The figure shows three views and two pictorial views of one solid part (mm, origin at its lowest corner). Answer the questions. A direction names the side the tool comes from. Give positions to 0.01 mm unless a question says otherwise; leave off trailing zeros. Order: outer loops, then holes, each group sorted by start corner. A loop starts at its lowest first (then second) coordinate and runs counter-clockwise, first axis right, second up. Notation, with made-up numbers: (49.25, 58.5) -> (62.25, 58.5) arc R18 ccw to (62.25, 91.5) -> close; hole circle Ø4 at (78.25, 54). An arc over 180 degrees is marked (long way). Use one line per item in the form item = value.
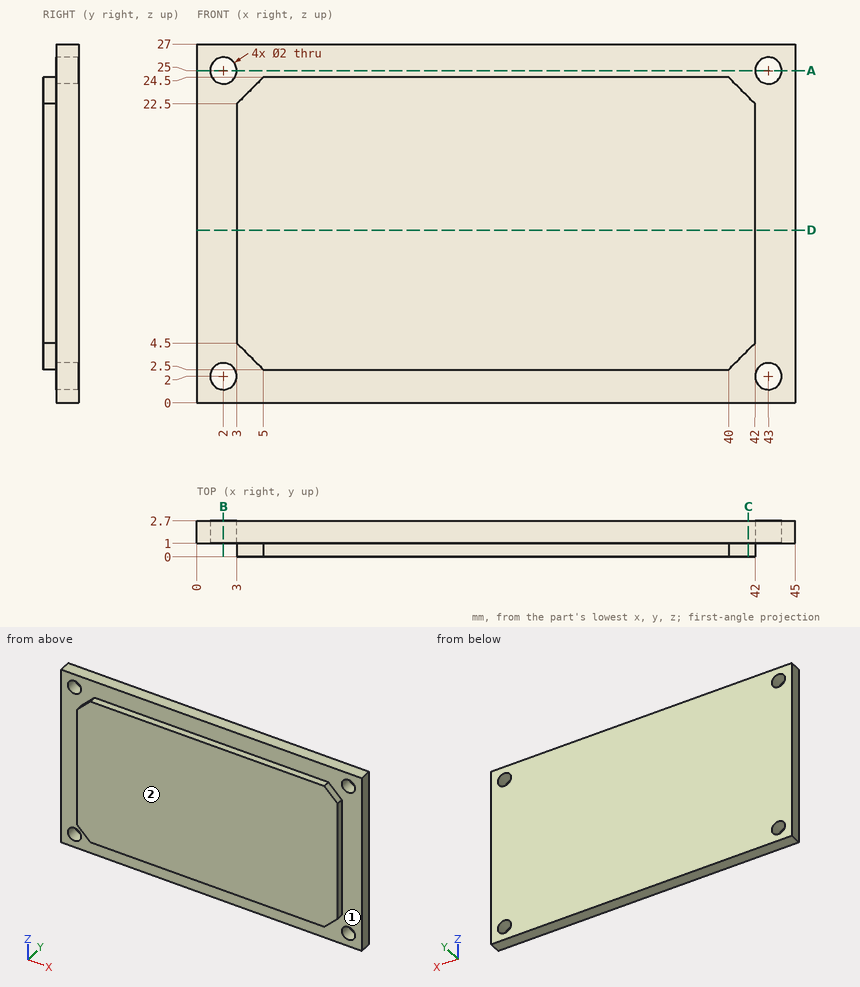
Item 1: The part is cut by section D-D on z = 13. Give the vertices of the cut face in (x, y).
Checks:
outline = (0, 1) -> (3, 1) -> (3, 0) -> (42, 0) -> (42, 1) -> (45, 1) -> (45, 2.7) -> (0, 2.7) -> close
Item 2: The part is cut by section B-B on x = 2. Give the vertices of the cut face in (y, z), and give its area (3 significant figures).
Checks:
outline = (1, 0) -> (2.7, 0) -> (2.7, 1) -> (1, 1) -> close; (1, 3) -> (2.7, 3) -> (2.7, 24) -> (1, 24) -> close; (1, 26) -> (2.7, 26) -> (2.7, 27) -> (1, 27) -> close
area = 39.1 mm²
Item 3: The part is cut by section A-A on z = 25. Give the vertices of the cut face in (x, y), and give its area (3 significant figures).
Checks:
outline = (0, 1) -> (1, 1) -> (1, 2.7) -> (0, 2.7) -> close; (3, 1) -> (42, 1) -> (42, 2.7) -> (3, 2.7) -> close; (44, 1) -> (45, 1) -> (45, 2.7) -> (44, 2.7) -> close
area = 69.7 mm²
Item 4: Given pin 1 Ø0.5 at (x, y) = (26.5, 0.5) entering from -Z; pin 2 Ø1.2 at (x, z) = (2, 2) entering from +Y; pin 3 Ø0.8 at (x, y) = (28.5, 0.5) entering from +Z; pin 4 Ø0.5 at (y, z) = (0.5, 18) entering from +X, each flat-ended and moving along its own axis, determine where each tip first touches the part or whether it passes through.
Checks:
pin_1 = 2.5
pin_2 = through
pin_3 = 24.5
pin_4 = 42
Item 5: The part is cut by section C-C on x = 41.5. Give the vertices of the cut face in (y, z).
Checks:
outline = (0, 4) -> (1, 4) -> (1, 0) -> (2.7, 0) -> (2.7, 27) -> (1, 27) -> (1, 23) -> (0, 23) -> close
Item 6: Straight lines are drawn through the part: L1, parallel to Z at x = 2, y = 2.3; L2, parallel to X at y = 0.65, z = 15; L3, parallel to Z at x = 27, y = 0.1. For each, find the intervals that lie inside material, in ascending order. Write a range as from..to.
Checks:
L1 = 0..1, 3..24, 26..27
L2 = 3..42
L3 = 2.5..24.5
Item 7: Which of the six approach directions +Z, -Z, +X, -X, +Y, -Y give full straight-line access (tool end or side, diameter ignored) to the marked faces 1 and 2?
Checks:
face_1 = -Y
face_2 = +Z, -Z, +X, -X, -Y
